The model under review builds one solid part; all positions refer to its coordinate system, in mm. A direction names the side the tool comes from. Round coordinates to 2 decimals unless told otherwise and drop trailing zeros. Loops run counter-clockwise (first coordinate to the right, second up) from the corner with the lowest first, then second, coordinate; pieces in that order, holes last. Notation, with made-up numbers: M 87.25,49.5 L 127.25,49.5 A3 cw 127.25,54.5 Z; hole C 25.25,-18.75 d10. An arc over 180 degrees is marked long. Answer in a Markdown table with one row per item. Add a question column.
from build123d import *

# Parameters (mm, degrees)
F0_R      = 9.4
F1_DEPTH  = 7
F2_R      = 2.5
F3_DEPTH  = 7
F4_R      = 1.25
F5_DEPTH  = 2.42
F6_R      = 2.25
F7_DEPTH  = 4.58
F8_R      = 1.45
F9_DEPTH  = 1.705
F10_R     = 2.2
F11_DEPTH = 5.295
F12_R     = 2.75
F13_DEPTH = 3
F15_DEPTH = 7


with BuildPart() as f1:
    # F0 (on Top) → F1 (new body)
    with BuildSketch(Plane.XY):
        Circle(F0_R)
    extrude(amount=F1_DEPTH)

    # F2 (on face) → F3 (join)
    with BuildSketch(Plane.XY.offset(7)):
        Circle(F2_R)
    extrude(amount=F3_DEPTH)

    # F4 (on face) → F5 (cut)
    with BuildSketch(Plane(origin=(0, 0, 0), x_dir=(1, 0, 0), z_dir=(0, 0, -1))):
        with Locations((6, 0)):
            Circle(F4_R)
        with Locations((-6, 0)):
            Circle(F4_R)
    extrude(amount=-F5_DEPTH, mode=Mode.SUBTRACT)

    # F6 (on face) → F7 (cut, through all)
    with BuildSketch(Plane(origin=(0, 0, 2.42), x_dir=(1, 0, 0), z_dir=(0, 0, -1))):
        with Locations((-6, 0)):
            Circle(F6_R)
        with Locations((6, 0)):
            Circle(F6_R)
    extrude(amount=-F7_DEPTH, mode=Mode.SUBTRACT)

    # F8 (on face) → F9 (cut)
    with BuildSketch(Plane(origin=(0, 0, 0), x_dir=(1, 0, 0), z_dir=(0, 0, -1))):
        with Locations((0, -6.5)):
            Circle(F8_R)
        with Locations((0, 6.5)):
            Circle(F8_R)
    extrude(amount=-F9_DEPTH, mode=Mode.SUBTRACT)

    # F10 (on face) → F11 (cut, through all)
    with BuildSketch(Plane(origin=(0, 0, 1.705), x_dir=(1, 0, 0), z_dir=(0, 0, -1))):
        with Locations((0, -6.5)):
            Circle(F10_R)
        with Locations((0, 6.5)):
            Circle(F10_R)
    extrude(amount=-F11_DEPTH, mode=Mode.SUBTRACT)

    # F12 (on face) → F13 (cut)
    with BuildSketch(Plane(origin=(0, 0, 0), x_dir=(1, 0, 0), z_dir=(0, 0, -1))):
        Circle(F12_R)
    extrude(amount=-F13_DEPTH, mode=Mode.SUBTRACT)

    # F14 (on face) → F15 (cut, through all)
    with BuildSketch(Plane.XY.offset(7)):
        with BuildLine():
            ThreePointArc((3.101538, -5.712308), (2.95297, -7.732869), (1.620693, -9.259231))
            ThreePointArc((1.620693, -9.259231), (7.197031, -6.046713), (9.4, 0))
            ThreePointArc((9.4, 0), (8.242264, -2.555827), (5.5575, -3.371082))
            Line((5.5575, -3.371082), (3.101538, -5.712308))
        make_face()
    extrude(amount=-F15_DEPTH, mode=Mode.SUBTRACT)


solid = f1.part
1. Take a section at B-B, the plane z = 5.75. State the section outline as (x, y) points, and give its area (3 significant figures).
2. Mouldability with a two-part tool opening along Y and no side actions: class faces 1 (the flat face through (-2.2, 2.2, 0)), 2 (the flat face through (0, 0, 3)), 3 (the cylindrical face through (-0.54, -2.44, 10.45)), 4 (the cylindrical face through (8.27, -2.53, 3.55)) as released by +Y, released by -Y, zero draft, split by the parting line, or undercut.
3. Take a section at D-D, the plane x = -6. State the section outline as (y, z) points.
4. For pin 1 Ø6 at (x, z) = (-0.5, 8.5) entering from +Y; pin 2 Ø2 at (x, y) = (6, 0) entering from +Z; pin 3 Ø4.5 at (x, y) = (0, 6.5) entering from +Z; pin 4 Ø1 at (x, z) = (0, 12.5) entering from +Y, all flat-tipped, find the tip position at first contact; note any pin that passes through.
5. Machinability: for faces 5 (the cylindrical face through (2.964, -7.706, 3.549)), 6 (the cylindrical face through (-0.596, 2.685, 1.479)), 7 (the flat face through (7, 1, 2.42)), which of the approach directions +Z, -Z, +X, -X, +Y, -Y give a long, thin tool a straight path to every point of the face, cutting with its end or side? Answer none if there is none.
6. Take a section at A-A, the plane x = 0. State the section outline as (y, z) points (3 decimals), and give its area (3 significant figures).
7. Take a section at C-C, the plane y = 6.25. State the section outline as (x, z) points (3 decimals), and give its area (3 significant figures).
8. To check wall thickness, follow probe 1 along Y at (x, z) = (0, 1.5); probe 2 along Y at (x, z) = (1.25, 4.75); probe 3 along Z at (x, y) = (-4, 5.25). State the ranges of each line that lie inside material, in increasing order.
Check sheet entries:
| question | item | result |
|---|---|---|
| 1 | outline | M 1.62,-9.26 A3.2 ccw 3.1,-5.71 L 5.56,-3.37 A3.4 ccw 9.4,0 A9.4 ccw long Z; hole C -6,0 d4.5; hole C 0,-6.5 d4.4; hole C 0,6.5 d4.4; hole C 6,0 d4.5 |
| 1 | area | 196 mm^2 |
| 2 | face 1 | zero draft |
| 2 | face 2 | undercut |
| 2 | face 3 | split by the parting line |
| 2 | face 4 | released by -Y |
| 3 | outline | M -7.24,0 L -1.25,0 L -1.25,2.42 L -2.25,2.42 L -2.25,7 L -7.24,7 Z; M 1.25,0 L 7.24,0 L 7.24,7 L 2.25,7 L 2.25,2.42 L 1.25,2.42 Z |
| 4 | pin 1 | stops at y = 9.4 |
| 4 | pin 2 | passes through |
| 4 | pin 3 | stops at z = 7 |
| 4 | pin 4 | stops at y = 2.5 |
| 5 | face 5 | +Z, -Z, +X |
| 5 | face 6 | -Z |
| 5 | face 7 | +Z |
| 6 | outline | M -9.4,0 L -7.95,0 L -7.95,1.705 L -8.7,1.705 L -8.7,7 L -9.4,7 Z; M -5.05,0 L -2.75,0 L -2.75,3 L 2.75,3 L 2.75,0 L 5.05,0 L 5.05,1.705 L 4.3,1.705 L 4.3,7 L 2.5,7 L 2.5,14 L -2.5,14 L -2.5,7 L -4.3,7 L -4.3,1.705 L -5.05,1.705 Z; M 7.95,0 L 9.4,0 L 9.4,7 L 8.7,7 L 8.7,1.705 L 7.95,1.705 Z |
| 6 | area | 93.6 mm^2 |
| 7 | outline | M -7.021,0 L -1.428,0 L -1.428,1.705 L -2.186,1.705 L -2.186,7 L -7.021,7 Z; M 1.428,0 L 7.021,0 L 7.021,7 L 2.186,7 L 2.186,1.705 L 1.428,1.705 Z |
| 7 | area | 70.3 mm^2 |
| 8 | probe 1 | y = -9.4 to -7.95, -5.05 to -2.75, 2.75 to 5.05, 7.95 to 9.4 |
| 8 | probe 2 | y = -9.32 to -8.31, -4.69 to 4.69, 8.31 to 9.32 |
| 8 | probe 3 | z = 0 to 7 |
